Verification items for the finished model (mm, model axes). Round coordinates to 2 decimals unless told otherwise and drop trailing zeros. Write each loop counter-clockwise with the first axis right and the second up, starting at its lowest first coordinate (ties: lowest second). Pieces come first, ordered by that corner, then holes.
from build123d import *

# Parameters (mm, degrees)
SKETCH1_W           = 304.8
SKETCH1_H           = 355.6
BOSS_EXTRUDE1_DEPTH = 1.5875


with BuildPart() as part:
    # Sketch1 → Boss-Extrude1 (new, symmetric)
    with BuildSketch(Plane(origin=(0, 0, 0), x_dir=(1, 0, 0), z_dir=(0, 1, 0))):
        Polygon((-152.4, -177.8), (-152.4, 177.8), (-254, 177.8), (-355.6, 177.8), (-355.6, -177.8), (-254, -177.8), align=None)
        Rectangle(SKETCH1_W, SKETCH1_H)
        Polygon((152.4, 177.8), (152.4, 279.4), (152.4, 381), (-152.4, 381), (-152.4, 279.4), (-152.4, 177.8), align=None)
        Polygon((152.4, -279.4), (152.4, -177.8), (-152.4, -177.8), (-152.4, -279.4), (-152.4, -381), (152.4, -381), align=None)
        Polygon((355.6, 177.8), (254, 177.8), (152.4, 177.8), (152.4, -177.8), (254, -177.8), (355.6, -177.8), align=None)
        Polygon((152.4, 177.8), (254, 177.8), (152.4, 279.4), align=None)
        Polygon((254, -177.8), (152.4, -177.8), (152.4, -279.4), align=None)
        Polygon((-152.4, -279.4), (-152.4, -177.8), (-254, -177.8), align=None)
        Polygon((-254, 177.8), (-152.4, 177.8), (-152.4, 279.4), align=None)
    extrude(amount=BOSS_EXTRUDE1_DEPTH, both=True)


solid = part.part
Q1. Sectioned sample at A-A (y = -0.3). Enter the section's corners in (x, z), plus the area to 3 significant figures.
Recorded:
outline: (-355.6, -177.8) - (-254, -177.8) - (-152.4, -279.4) - (-152.4, -381) - (152.4, -381) - (152.4, -279.4) - (254, -177.8) - (355.6, -177.8) - (355.6, 177.8) - (254, 177.8) - (152.4, 279.4) - (152.4, 381) - (-152.4, 381) - (-152.4, 279.4) - (-254, 177.8) - (-355.6, 177.8) - close
area: 397,000 mm2
Q2. Depth check by flat-ended pin: P1, Ø1.6, axis at y = 0, z = 334, coming from the +X side; P2, Ø1.6, axis at x = -299.5, y = 0, coming from the +Z side. Enter the tip coordinate at first touch or a pass-through.
Recorded:
P1: stops at x = 152.4
P2: stops at z = 177.8
Q3. Sectioned sample at B-B (x = 176). Enter the section's corners in (y, z), plus the area to 3 significant figures.
Recorded:
outline: (-1.59, -255.8) - (1.59, -255.8) - (1.59, 255.8) - (-1.59, 255.8) - close
area: 1,620 mm2
Q4. Sectioned sample at C-C (z = -247.5). Enter the section's corners in (x, y), plus the area to 3 significant figures.
Recorded:
outline: (-184.3, -1.59) - (184.3, -1.59) - (184.3, 1.59) - (-184.3, 1.59) - close
area: 1,170 mm2
Q5. Material ranges on line 1 along X through (y, z) = (-0.4, -311.5); line 2 along Z through (x, y) = (283.5, 0.9); line 3 along Z through (x, y) = (161.5, 0.7), recorded low to high.
Recorded:
line 1: x = -152.4 to 152.4
line 2: z = -177.8 to 177.8
line 3: z = -270.3 to 270.3
